Here's how the part is built. I have some questions about the finished solid (model axes, mm). A direction names the side the tool comes from. Round coordinates to 2 decimals unless told otherwise and drop trailing zeros. Loops run counter-clockwise (first coordinate to the right, second up) from the corner with the lowest first, then second, coordinate; pieces in that order, holes last. Notation, with made-up numbers: (41, 22.25) -> (55, 22.25) arc R17 ccw to (55, 44.25) -> close; hole circle Ø11 at (-8.75, 36.25). An arc over 180 degrees is marked (long way). Use one line per item in the form item = value. Start each with the question number.
Item 1: I'm going to push flat-ended pins straight in: pin 1 Ø10 at (y, z) = (-28.5, 25.5) entering from +X; pin 2 Ø4 at (y, z) = (-5, 3.5) entering from +X; pin 3 Ø9 at (x, z) = (25.5, 22) entering from -Y. Where does each tip first touch, or does it pass through?
Item 2: If we section it at D-D (x = 27): Write out the boundary of the cut face in (y, z).
Item 3: If I drill on L1, parallel to Z at x = -2, y = -27; L2, parallel to Z at x = -1.65, y = -13; L3, parallel to X at y = -11, z = 19.5, over which ranges is the centre line in solid material (lowest first)? Write a range as [from, to].
Item 4: If we section it at A-A (x = 13): Write out the boundary of the cut face in (y, z), then the cut area to 3 significant figures.
Item 5: For faces 4 (the face through (0, -20, 15)), 5 (the face through (-2.317, -14.524, 14.368)), which set-ups out of +Z, -Z, +X, -X, +Y, -Y let a thin tool reach every point of the face, with its end or its side?
Item 6: Thinking about a two-plate mould opening in X: for faces 1 (the face through (-1, -8, 0)), 2 (the face through (28.216, 2.317, 23.115)), 3 (the face through (-0.507, -37.193, 14.79)), which applies, released by +X, released by -X, zero draft, split by the parting line, or undercut?
Item 7: If we section it at B-B (y = -13): Write out the boundary of the cut face in (x, z), then the cut area to 3 significant figures.
Item 8: If we section it at C-C (z = 22): State how many separate pieces and enclosed holes the cut face has, then the cut area to 3 significant figures.
```python
from build123d import *

# Parameters (mm, degrees)
F1_DEPTH             = 30
F4_D                 = 3.3
F4_CSINK_D           = 5.5
F4_CSINK_ANGLE       = 90
F4_ON_F3_D           = 3.3
F4_ON_F3_CSINK_D     = 5.5
F4_ON_F3_CSINK_ANGLE = 90
F5_R                 = 1


with BuildPart() as f1:
    # F0 (on Top) → F1 (new body)
    with BuildSketch(Plane.XY):
        with BuildLine():
            ThreePointArc((-3.5, -39.7696960071), (-0.9688711259, -37.9580398915), (0, -35))
            Line((0, -35), (0, -5))
            ThreePointArc((0, -5), (1.4644660941, -1.4644660941), (5, 0))
            Line((5, 0), (35, 0))
            ThreePointArc((35, 0), (37.9580398915, 0.9688711259), (39.7696960071, 3.5))
            Line((39.7696960071, 3.5), (-1.5, 3.5))
            ThreePointArc((-1.5, 3.5), (-2.9142135624, 2.9142135624), (-3.5, 1.5))
            Line((-3.5, 1.5), (-3.5, -39.7696960071))
        make_face()
    extrude(amount=F1_DEPTH)

    # F4 (through all)
    with Locations(Plane.XZ):
        with Locations((13, 15), (27, 22), (27, 8)):
            CounterSinkHole(F4_D / 2, F4_CSINK_D / 2, counter_sink_angle=F4_CSINK_ANGLE)

    # F4 on F3 (through all)
    with Locations(Plane.YZ):
        with Locations((-13, 15), (-27, 22), (-27, 8)):
            CounterSinkHole(F4_ON_F3_D / 2, F4_ON_F3_CSINK_D / 2, counter_sink_angle=F4_ON_F3_CSINK_ANGLE)

    # F5
    f5_edges = [f1.edges().sort_by_distance(p)[0] for p in [
        (-3.5, -39.769696, 15),
        (39.769696, 3.5, 15),
    ]]
    fillet(f5_edges, radius=F5_R)


solid = f1.part
```
Values found:
q1.pin_1 = 0
q1.pin_2 = 0.42
q1.pin_3 = 0
q2.outline = (0, 0) -> (3.5, 0) -> (3.5, 6.35) -> (1.1, 6.35) -> (0, 5.25) -> close; (0, 10.75) -> (1.1, 9.65) -> (3.5, 9.65) -> (3.5, 20.35) -> (1.1, 20.35) -> (0, 19.25) -> close; (0, 24.75) -> (1.1, 23.65) -> (3.5, 23.65) -> (3.5, 30) -> (0, 30) -> close
q3.L1 = [0, 6.35], [9.65, 20.35], [23.65, 30]
q3.L2 = [0, 13.35], [16.65, 30]
q3.L3 = [-3.5, 0]
q4.outline = (0, 0) -> (3.5, 0) -> (3.5, 13.35) -> (1.1, 13.35) -> (0, 12.25) -> close; (0, 17.75) -> (1.1, 16.65) -> (3.5, 16.65) -> (3.5, 30) -> (0, 30) -> close
q4.area = 92.2 mm2
q5.face_4 = +Z, -Z, +X, -Y
q5.face_5 = +X, -X
q6.face_1 = zero draft
q6.face_2 = undercut
q6.face_3 = released by +X
q7.outline = (-3.5, 0) -> (0, 0) -> (0, 12.25) -> (-1.1, 13.35) -> (-3.5, 13.35) -> close; (-3.5, 16.65) -> (-1.1, 16.65) -> (0, 17.75) -> (0, 30) -> (-3.5, 30) -> close
q7.area = 92.2 mm2
q8.separate_pieces = 3
q8.enclosed_holes = 0
q8.area = 259 mm2
